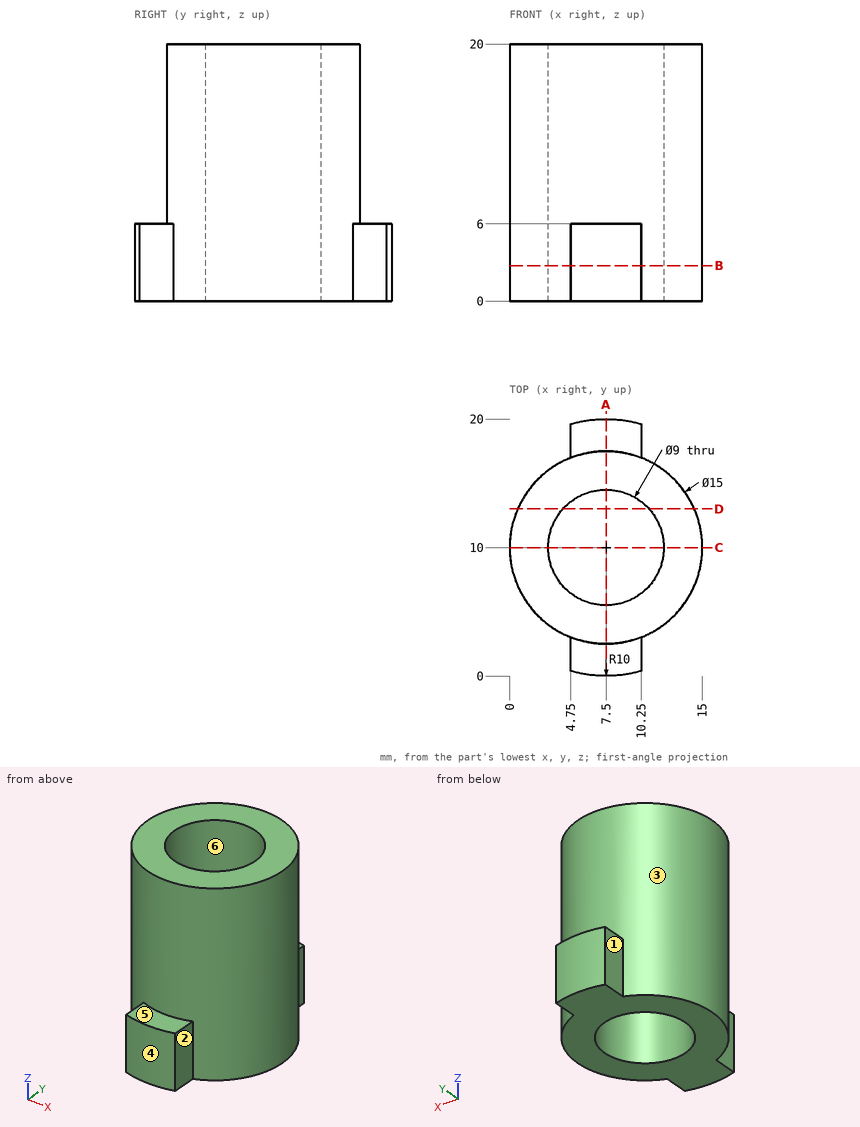
Geometry: see drawing. Coordinates: mm, zero at the bounding-box minimum. A direction names the side the tool comes from. Coordinates: 2 decimals unless noted, no trailing zeros. Loops run counter-clockwise (first coordinate to the right, second up) from the corner with the lowest first, then second, coordinate; pieces in that order, holes last. Notation, with made-up numbers: M 39.25,-0.75 L 63.25,-0.75 A21 cw 63.25,15.25 Z; hole C 84,42.5 d4. An arc over 180 degrees is marked long. Answer in a Markdown table with one row per item.
1. Reachability of the marked faces 1, 2 and 3 from +Z, -Z, +X, -X, +Y, -Y: full face, straight path, thin tool, end or side. Return the list, or none.
Response:
| item | result |
|---|---|
| face 1 | +Z, -Z, -X, +Y |
| face 2 | +Z, -Z, +X, -Y |
| face 3 | +Z |
2. Section D-D, the plane y = 13. Output: boundary loops of the cut face in (x, z).
Response:
| item | result |
|---|---|
| outline | M 0.63,0 L 4.15,0 L 4.15,20 L 0.63,20 Z; M 10.85,0 L 14.37,0 L 14.37,20 L 10.85,20 Z |
3. Section C-C, the plane y = 10. Output: boundary loops of the cut face in (x, z), then the cut area to 3 significant figures.
Response:
| item | result |
|---|---|
| outline | M 0,0 L 3,0 L 3,20 L 0,20 Z; M 12,0 L 15,0 L 15,20 L 12,20 Z |
| area | 120 mm2 |
4. Section A-A, the plane x = 7.5. Output: boundary loops of the cut face in (y, z), then the cut area to 3 significant figures.
Response:
| item | result |
|---|---|
| outline | M 0,0 L 5.5,0 L 5.5,20 L 2.5,20 L 2.5,6 L 0,6 Z; M 14.5,0 L 20,0 L 20,6 L 17.5,6 L 17.5,20 L 14.5,20 Z |
| area | 150 mm2 |
5. First-contact query: pin 1 (1.3 mm diameter, centred on y = 1, z = 4, fed in from +X); pin 2 (1.3 mm diameter, centred on y = 18, z = 4, fed in from -X); pin 3 (4 mm diameter, centred on y = 7.5, z = 16.5, fed in from -X); pin 4 (7 mm diameter, centred on x = 7.5, y = 10, fed in from -Z). Flat tips, straight axial feed; report the tip coordinate or a pass-through.
Response:
| item | result |
|---|---|
| pin 1 | stops at x = 10.25 |
| pin 2 | stops at x = 4.75 |
| pin 3 | stops at x = 0.02 |
| pin 4 | passes through |
6. Section B-B, the plane z = 2.75. Output: boundary loops of the cut face in (x, y), then the cut area to 3 significant figures.
Response:
| item | result |
|---|---|
| outline | M 4.75,0.39 A10 ccw 10.25,0.39 L 10.25,3.02 A7.5 ccw 10.25,16.98 L 10.25,19.61 A10 ccw 4.75,19.61 L 4.75,16.98 A7.5 ccw 4.75,3.02 Z; hole C 7.5,10 d9 |
| area | 141 mm2 |
7. Material intervals for line 1 (Y direction, x = 7.5, z = 15); line 2 (Y direction, x = 3.5, z = 7.5); line 3 (Y direction, x = 13.5, z = 17.5), sorted ascending.
Response:
| item | result |
|---|---|
| line 1 | y = 2.5 to 5.5, 14.5 to 17.5 |
| line 2 | y = 3.66 to 7.94, 12.06 to 16.34 |
| line 3 | y = 5.5 to 14.5 |
8. Draft query along X for the marked faces 4, 5 and 6. Return one class per face: pulls with the +X half, pulls with the -X half, needs draft (parallel to the pull), parting line crosses it, or undercut.
Response:
| item | result |
|---|---|
| face 4 | parting line crosses it |
| face 5 | needs draft |
| face 6 | undercut |
